The listing builds one solid part. Answer for the finished solid, in the listing's coordinates (mm). A direction names the side the tool comes from. Round coordinates to 2 decimals unless told otherwise and drop trailing zeros. Order: outer loops, then holes, each group sorted by start corner. A loop starts at its lowest first (then second) coordinate and runs counter-clockwise, first axis right, second up. Notation, with made-up numbers: (63.25, -39.75) -> (111.25, -39.75) arc R26 ccw to (111.25, -9.75) -> close; hole circle Ø8 at (43, 33.5). An arc over 180 degrees is marked (long way). Answer in a Markdown table with one row per item. Add a question column.
```python
from build123d import *

# Parameters (mm, degrees)
F1_DEPTH = 2
F2_DEPTH = 7
F3_R     = 2.99999


# Not quite as in the source:
# - a fillet or chamfer is up to 0.001 mm smaller than in the source, because OpenCascade refuses the exact size


with BuildPart() as f1:
    # F0 (on Top) → F1 (new body)
    with BuildSketch(Plane.XY):
        Polygon((15.7818826017, 10.0030450644), (-10.2181173983, 10.0030450644), (-10.2181173983, -15.9969549356), (-8.2181173983, -15.9969549356), (-8.2181173983, 8.0030450644), (15.7818826017, 8.0030450644), align=None)
        Polygon((15.7818826017, 6.0030450644), (15.7818826017, 8.0030450644), (-8.2181173983, 8.0030450644), (-8.2181173983, -15.9969549356), (-6.2181173983, -15.9969549356), (-6.2181173983, 6.0030450644), align=None)
        Polygon((15.7818826017, 4.0030450644), (15.7818826017, 6.0030450644), (-6.2181173983, 6.0030450644), (-6.2181173983, -15.9969549356), (-4.2181173983, -15.9969549356), (-4.2181173983, 4.0030450644), align=None)
        Polygon((17.7818826017, 10.0030450644), (15.7818826017, 10.0030450644), (15.7818826017, 8.0030450644), (15.7818826017, 6.0030450644), (15.7818826017, 4.0030450644), (17.7818826017, 4.0030450644), align=None)
        Polygon((-8.2181173983, -15.9969549356), (-10.2181173983, -15.9969549356), (-10.2181173983, -17.9969549356), (-4.2181173983, -17.9969549356), (-4.2181173983, -15.9969549356), (-6.2181173983, -15.9969549356), align=None)
    extrude(amount=-F1_DEPTH)

    # F0 (on Top) → F2 (join)
    with BuildSketch(Plane.XY):
        Polygon((15.7818826017, 10.0030450644), (-10.2181173983, 10.0030450644), (-10.2181173983, -15.9969549356), (-8.2181173983, -15.9969549356), (-8.2181173983, 8.0030450644), (15.7818826017, 8.0030450644), align=None)
        Polygon((15.7818826017, 4.0030450644), (15.7818826017, 6.0030450644), (-6.2181173983, 6.0030450644), (-6.2181173983, -15.9969549356), (-4.2181173983, -15.9969549356), (-4.2181173983, 4.0030450644), align=None)
        Polygon((17.7818826017, 10.0030450644), (15.7818826017, 10.0030450644), (15.7818826017, 8.0030450644), (15.7818826017, 6.0030450644), (15.7818826017, 4.0030450644), (17.7818826017, 4.0030450644), align=None)
        Polygon((-8.2181173983, -15.9969549356), (-10.2181173983, -15.9969549356), (-10.2181173983, -17.9969549356), (-4.2181173983, -17.9969549356), (-4.2181173983, -15.9969549356), (-6.2181173983, -15.9969549356), align=None)
    extrude(amount=F2_DEPTH)

    # F3 (radius 3 in the source; OpenCascade refuses exactly that, so slightly less here)
    f3_edges = [f1.edges().sort_by_distance(p)[0] for p in [
        (-4.218117, 4.003045, 2.5),
        (-10.218117, 10.003045, 2.5),
        (-10.218117, -17.996955, 2.5),
        (-4.218117, -17.996955, 2.5),
        (17.781883, 4.003045, 2.5),
        (17.781883, 10.003045, 2.5),
    ]]
    fillet(f3_edges, radius=F3_R)


solid = f1.part
```
1. The mould has two halves that part along X. Classify faces 1 (the flat face through (5, 6.003, 3)), 2 (the cylindrical face through (16.93, 4.91, 2.44)), 3 (the flat face through (4, 10.003, 2)): released by +X, released by -X, zero draft, split by the parting line, or undercut.
2. The part is cut by section B-B (x = 9.5). Give the vertices of the cut face in (y, z).
3. For faces 4 (the flat face through (7, 4.003, 2)), 5 (the flat face through (-7, -15.997, 3)), 6 (the cylindrical face through (-9.363, -17.095, 2.563)), determine the directions among +Z, -Z, +X, -X, +Y, -Y from which every point of the face is accessible in a straight line to the end or side of a thin tool.
4. The part is cut by section C-C (y = -7.75). Give the vertices of the cut face in (x, z), then the cut area to 3 significant figures.
5. Each of these flat-tipped pins is pushed along its axis until it touches: pin 1 (12 mm diameter, centred on x = 3.5, y = -2.5, fed in from +Z); pin 2 (2.5 mm diameter, centred on x = 9, z = 2, fed in from -Y). Where does it stop, or does it pass through?
6. Straight lines are drawn through the part: line 1 along X through (y, z) = (-12.25, 4.5); line 2 along Y through (x, z) = (14.25, 2.5); line 3 along Y through (x, z) = (-7, 4.5). For each, find the intervals that lie inside material, in ascending order.
Report:
| question | item | result |
|---|---|---|
| 1 | face 1 | undercut |
| 1 | face 2 | released by +X |
| 1 | face 3 | zero draft |
| 2 | outline | (4, -2) -> (10, -2) -> (10, 7) -> (8, 7) -> (8, 0) -> (6, 0) -> (6, 7) -> (4, 7) -> close |
| 3 | face 4 | +Z, -Z, +X, -Y |
| 3 | face 5 | +Z |
| 3 | face 6 | +Z, -Z, -X, -Y |
| 4 | outline | (-10.22, -2) -> (-4.22, -2) -> (-4.22, 7) -> (-6.22, 7) -> (-6.22, 0) -> (-8.22, 0) -> (-8.22, 7) -> (-10.22, 7) -> close |
| 4 | area | 40.0 mm^2 |
| 5 | pin 1 | passes through |
| 5 | pin 2 | stops at y = 4 |
| 6 | line 1 | x = -10.22 to -8.22, -6.22 to -4.22 |
| 6 | line 2 | y = 4 to 6, 8 to 10 |
| 6 | line 3 | y = -17.99 to -16, 8 to 10 |
